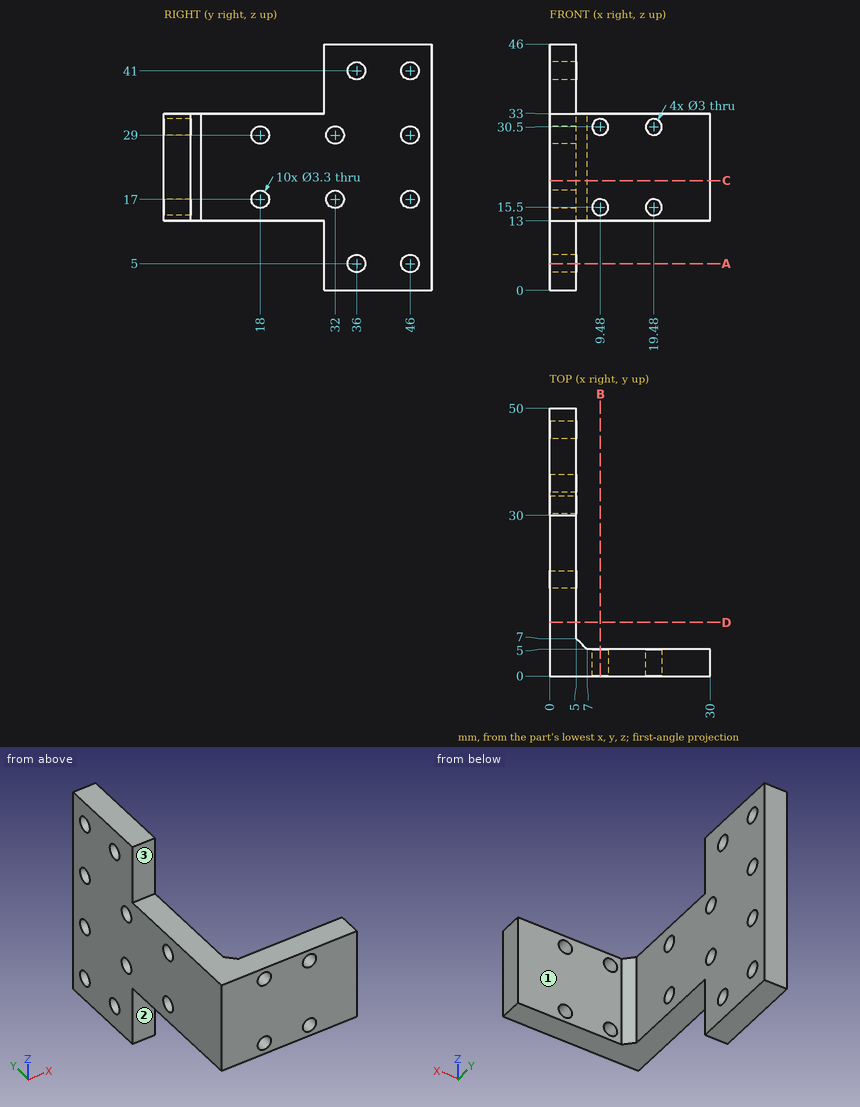
Can you work these out from the drawing? Everything is in mm from the part's minimum corner. A direction names the side the tool comes from. Round coordinates to 2 decimals unless told otherwise and drop trailing zeros. Loops run counter-clockwise (first coordinate to the right, second up) from the corner with the lowest first, then second, coordinate; pieces in that order, holes last. Notation, with made-up numbers: (2.5, 1.5) - (10.5, 1.5) arc R5 cw to (10.5, 10.5) - close; hole circle Ø6 at (-13.75, 7.5). An arc over 180 degrees is marked (long way). Answer in a Markdown table with one row per item. Add a question column.
Q1. For pin 1 Ø10 at (x, z) = (20, 17) entering from -Y; pin 2 Ø13 at (y, z) = (26, 33.5) entering from +X; pin 3 Ø5 at (x, z) = (19.48, 30.5) entering from +Y, each with a flat end and sliding along its axis, tell me the tip position at first contact or that it passes through.
Q2. I need wall thicknesses on L1, parallel to Z at x = 19.48, y = 2.55; L2, parallel to Z at x = 1.05, y = 32; L3, parallel to Y at x = 3.35, z = 5. Which ranges of each line are inside material? Lowest first, please.
Q3. I want a section at C-C on z = 20.5. List the corners of the cut face in (x, y) for me, and give its area (3 significant figures).
Q4. Which directions (+Z, -Z, +X, -X, +Y, -Y) give clear straight access to the entire face, cutting with the end or side of a thin tool? Please do the marked faces 1, 2 and 3.
Q5. I want a section at D-D on y = 10. List the corners of the cut face in (x, z) for me, and give its area (3 significant figures).
Q6. I want a section at B-B on x = 9.48. List the corners of the cut face in (y, z) for me, and give its area (3 significant figures).
Q7. I want a section at A-A on z = 5. List the corners of the cut face in (x, y) for me.
A:
| question | item | result |
|---|---|---|
| 1 | pin 1 | y = 0 |
| 1 | pin 2 | x = 5 |
| 1 | pin 3 | y = 5 |
| 2 | L1 | 13 to 14, 17 to 29, 32 to 33 |
| 2 | L2 | 0 to 15.35, 18.65 to 27.35, 30.65 to 46 |
| 2 | L3 | 30 to 34.35, 37.65 to 44.35, 47.65 to 50 |
| 3 | outline | (0, 0) - (30, 0) - (30, 5) - (7, 5) - (5, 7) - (5, 50) - (0, 50) - close |
| 3 | area | 377 mm^2 |
| 4 | face 1 | +Z, -Z, +X, +Y |
| 4 | face 2 | -Z, +X, -X, -Y |
| 4 | face 3 | +Z, +X, -X, -Y |
| 5 | outline | (0, 13) - (5, 13) - (5, 33) - (0, 33) - close |
| 5 | area | 100 mm^2 |
| 6 | outline | (0, 13) - (5, 13) - (5, 14) - (0, 14) - close; (0, 17) - (5, 17) - (5, 29) - (0, 29) - close; (0, 32) - (5, 32) - (5, 33) - (0, 33) - close |
| 6 | area | 70.0 mm^2 |
| 7 | outline | (0, 30) - (5, 30) - (5, 34.35) - (0, 34.35) - close; (0, 37.65) - (5, 37.65) - (5, 44.35) - (0, 44.35) - close; (0, 47.65) - (5, 47.65) - (5, 50) - (0, 50) - close |
